Source: CAD feature listing. Evaluate the final solid. Frame: model axes, mm. Round coordinates to 2 decimals unless told otherwise and drop trailing zeros. Loops run counter-clockwise (first coordinate to the right, second up) from the corner with the lowest first, then second, coordinate; pieces in that order, holes last. Notation, with made-up numbers: M 60.25,71 L 64.25,71 A22 cw 64.25,98 Z; hole C 84,58 d7. An arc over 180 degrees is marked long. One line per item, written item: value.
from build123d import *

# Parameters (mm, degrees)
SKIZZE1_W                       = 250
SKIZZE1_H                       = 250
AUFSATZ_LINEAR_AUSTRAGEN1_DEPTH = 2
SKIZZE2_R                       = 3
SCHNITT_LINEAR_AUSTRAGEN1_DEPTH = 3
M4_GEWINDEBOHRUNG1_D            = 3.3


with BuildPart() as part:
    # Skizze1 → Aufsatz-Linear austragen1 (new body)
    with BuildSketch(Plane.XY):
        Rectangle(SKIZZE1_W, SKIZZE1_H)
    extrude(amount=AUFSATZ_LINEAR_AUSTRAGEN1_DEPTH)

    # Skizze2 → Schnitt-Linear austragen1 (cut, through all)
    with BuildSketch(Plane.XY.offset(2)):
        with Locations((0, 85)):
            Circle(SKIZZE2_R)
        with Locations((-50, 85)):
            Circle(SKIZZE2_R)
        with Locations((50, 85)):
            Circle(SKIZZE2_R)
    extrude(amount=-SCHNITT_LINEAR_AUSTRAGEN1_DEPTH, mode=Mode.SUBTRACT)

    # M4 Gewindebohrung1 (through all)
    with Locations(Plane(origin=(0, 0, 0), x_dir=(-1, 0, 0), z_dir=(0, 0, -1))):
        with Locations((-80, -117.64), (-50, -117.64), (-20, -117.64), (10, -117.64), (40, -117.64), (70, -117.64), (100, -117.64)):
            Hole(M4_GEWINDEBOHRUNG1_D / 2)


solid = part.part
1. Section query A-A (y = 85). Return the cut outline in (x, z), and give its area (3 significant figures).
Report:
outline: M -125,0 L -53,0 L -53,2 L -125,2 Z; M -47,0 L -3,0 L -3,2 L -47,2 Z; M 3,0 L 47,0 L 47,2 L 3,2 Z; M 53,0 L 125,0 L 125,2 L 53,2 Z
area: 464 mm2
2. Section query B-B (x = 0). Return the cut outline in (y, z), and give its area (3 significant figures).
Report:
outline: M -125,0 L 82,0 L 82,2 L -125,2 Z; M 88,0 L 125,0 L 125,2 L 88,2 Z
area: 488 mm2
3. Ray query, line 1 (Y direction, x = 50, z = 1.3); line 2 (Y direction, x = -40, z = 0.8); line 3 (X direction, y = 82.5, z = 0.65). Return the intervals inside material, ascending. Write a range as [from, to].
Report:
line 1: y = [-125, -119.29], [-115.99, 82], [88, 125]
line 2: y = [-125, -119.29], [-115.99, 125]
line 3: x = [-125, -51.66], [-48.34, -1.66], [1.66, 48.34], [51.66, 125]
4. Pull-direction query (X, two-part tool) for faces 1 (the face through (49.35, 82.07, 1.01)), 2 (the face through (-2, 2, 2)); classes: released by +X, released by -X, zero draft, split by the parting line, or undercut.
Report:
face 1: undercut
face 2: zero draft
5. Pin query (flat end, axial travel): pin 1 (4.5 mm diameter, centred on x = 80, y = -117.64, fed in from +Z). Return the tip coordinate at first contact, or that it passes through.
Report:
pin 1: stops at z = 2
